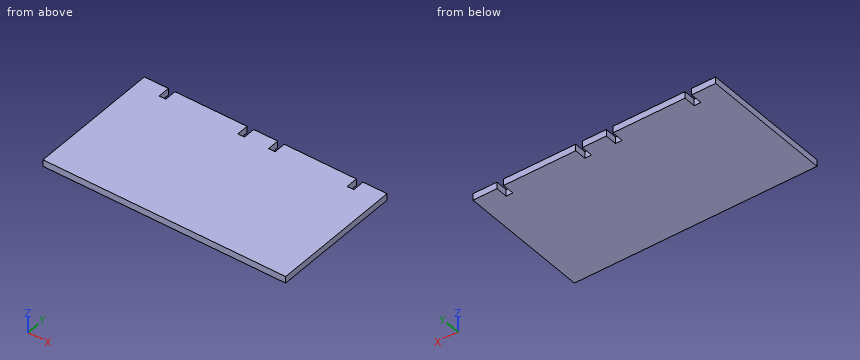
Autodesk Inventor part; units mm, degrees
ref_plane "YZ Plane" through (0, 0, 0) normal (1, 0, 0) x (0, 1, 0)
ref_plane "XZ Plane" through (0, 0, 0) normal (0, 1, 0) x (-1, 0, 0)
ref_plane "XY Plane" through (0, 0, 0) normal (0, 0, 1) x (1, 0, 0)
sketch "Sketch2" plane through (0, 0, 0) normal (0, 0, 1) x (1, 0, 0)
  line L0 (0, 0) -> (106.5, 0)
  line L1 (106.5, 0) -> (106.5, 110) construction
  line L2 (106.5, 110) -> (0, 110)
  line L3 (0, 110) -> (0, 0)
  line L4 (213, 0) -> (106.5, 0)
  line L5 (106.5, 110) -> (213, 110)
  line L6 (213, 110) -> (213, 0)
  line L7 (5.5, 100) -> (5.5, 110)
  line L8 (5.5, 110) -> (0, 110)
  line L9 (0, 110) -> (0, 100)
  line L10 (0, 100) -> (5.5, 100)
  line L11 (5.5, 100) -> (0, 110) construction
  line L12 (5.5, 110) -> (0, 100) construction
  line L13 (213, 100) -> (207.5, 100)
  line L14 (207.5, 100) -> (207.5, 110)
  line L15 (207.5, 110) -> (213, 110)
  line L16 (207.5, 100) -> (213, 110) construction
  line L17 (207.5, 110) -> (213, 100) construction
  line L18 (213, 110) -> (213, 100)
  line L19 (106.5, 0.9442) -> (106.5, 183.5442) construction
  line L20 (31, 100) -> (31, 110)
  line L21 (25.5, 110) -> (25.5, 100)
  line L22 (25.5, 100) -> (31, 100)
  line L23 (31, 100) -> (25.5, 110) construction
  line L24 (31, 110) -> (25.5, 100) construction
  line L25 (96.5, 100) -> (96.5, 110)
  line L26 (91, 110) -> (91, 100)
  line L27 (91, 100) -> (96.5, 100)
  line L28 (96.5, 100) -> (91, 110) construction
  line L29 (96.5, 110) -> (91, 100) construction
  line L30 (122, 100) -> (116.5, 100)
  line L31 (116.5, 100) -> (116.5, 110)
  line L32 (116.5, 100) -> (122, 110) construction
  line L33 (116.5, 110) -> (122, 100) construction
  line L34 (122, 110) -> (122, 100)
  line L35 (187.5, 100) -> (182, 100)
  line L36 (182, 100) -> (182, 110)
  line L37 (182, 110) -> (187.5, 100) construction
  line L38 (182, 100) -> (187.5, 110) construction
  line L39 (187.5, 110) -> (187.5, 100)
  line L40 (28.25, 105) -> (93.75, 105) construction
  line L41 (5.5, 100) -> (5.5, 0)
  line L42 (207.5, 100) -> (207.5, 0)
  point P0 (0, 100)
  point P1 (119.25, 105)
  point P2 (184.75, 105)
  point P3 (182, 110)
  point P4 (31, 110)
  point P5 (25.5, 110)
  dimension "d18" = 106.5
  dimension "d19" = 5.5
  dimension "d30" = 10
  dimension "d33" = 100
  dimension "d38" = 10
  dimension "d47" = 20
extrude "Extrusion3" add sketch "Sketch2" along normal blind 5.5 contours L41 L7 L2 L21 L22 L20 L26 L27 L25 L5 L31 L30 L34 L36 L35 L39 L14 L42 L4 L0
equation "\"d38\" = 0.5 * d43"
equation "\"d47\" = lrbottomw"
equation "\"thick\" = 0.5"
equation "\"lrlr\" = 19"
equation "\"lrmid\" = 19.9"
equation "\"lrdepth\" = 3.3"
equation "\"mlr\" = 16.6"
equation "\"mmid\" = 24.7"
equation "\"mdepth\" = 4.5"
equation "\"lrltotal\" = 126.6"
equation "\"mltotal\" = 126.6"
equation "\"lrbetween\" = 52.1"
equation "\"mbetween\" = 49.5"
equation "\"toler\" = 1"
equation "\"lrbottomw\" = 20"
equation "\"tight\" = 0.08"
equation "\"stuckw\" = 6"
equation "\"sidewallL\" = 132.6"
equation "\"heaterH\" = 117.3"
equation "\"stickL\" = 3.5"
equation "\"wireH\" = 25"
properties part number "wire_bottom"
The listing builds one solid part. Answer for the finished solid, in the listing's coordinates (mm). Coordinates: 2 decimals unless noted, no trailing zeros. Write each loop counter-clockwise with the first axis right and the second up, starting at its lowest first coordinate (ties: lowest second). Pieces come first, ordered by that corner, then holes. Notation, with made-up numbers: (25, -15) -> (50, -15) arc R21 ccw to (50, -4) -> close; hole circle Ø9 at (52, 11.25). An arc over 180 degrees is marked (long way). One line per question, with ' | ' between items.
1. Section A-A (x = 184) is taken. Determine the outline of the cut face in (y, z), and give its area (3 significant figures).
Verdict:
outline: (0, 0) -> (100, 0) -> (100, 5.5) -> (0, 5.5) -> close | area: 550 mm^2
2. Given pin 1 Ø1.6 at (x, z) = (185, 2.5) entering from +Y, flat-ended and moving along its own axis, determine where the tip first touches the part or whether it passes through.
Verdict:
pin 1: stops at y = 100
3. Straight lines are drawn through the part: line 1 (X direction, y = 104.5, z = 2); line 2 (Y direction, x = 187, z = 5.15). For each, find the intervals that lie inside material, in ascending order.
Verdict:
line 1: x = 5.5 to 25.5, 31 to 91, 96.5 to 116.5, 122 to 182, 187.5 to 207.5 | line 2: y = 0 to 100
